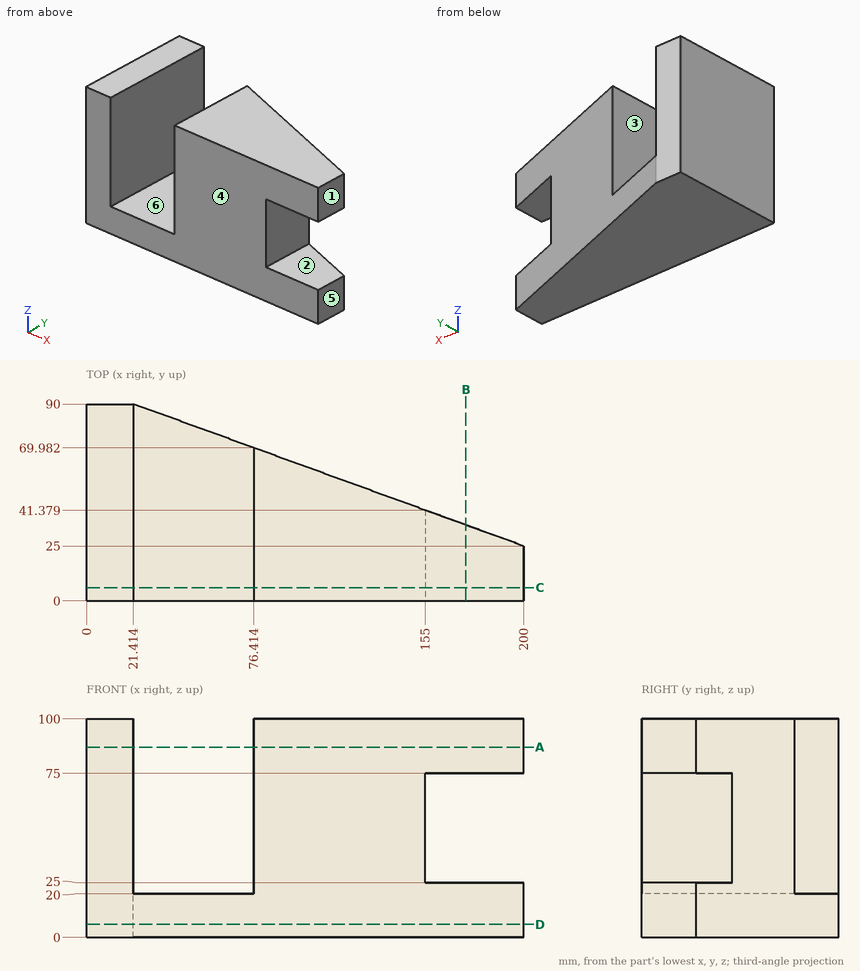
Here's the drawing with two shaded views (mm, measured from the low corner). I have some questions. A direction names the side the tool comes from. Coordinates: 2 decimals unless noted, no trailing zeros. Write each loop counter-clockwise with the first axis right and the second up, starting at its lowest first coordinate (ties: lowest second). Pieces come first, ordered by that corner, then holes.
Item 1: If I drill on line 1 (X direction, y = 8, z = 66); line 2 (Z direction, x = 162, y = 29.5); line 3 (Z direction, x = 45, y = 12.5), over which ranges is the centre line in solid material (lowest first)?
Item 2: I want a section at C-C on y = 6. Write out the boundary of the cut face in (x, z), and give its area (4 significant figures).
Item 3: If we mould it in two halves opening along X, with no side actions, what happens to the marked faces 4, 5 and 6? For each: +X half, -X half, draft (parallel to the pull), parting line (faces both ways), or undercut.
Item 4: I want a section at B-B on x = 173.5. Write out the boundary of the cut face in (y, z) (1 decimal).
Item 5: Will these pins go through, and if not, where does the flat tip stop? pin 1 (8 mm diameter, centred on x = 62, z = 20.5, fed in from +Y); pin 2 (12.5 mm diameter, centred on y = 19.5, z = 56, fed in from +X); pin 3 (5 mm diameter, centred on x = 66.5, y = 57.5, fed in from +Z).
Item 6: I want a section at A-A on z = 87. Write out the boundary of the cut face in (x, y), and give its area (3 significant figures).
Item 7: I want a section at D-D on z = 6. Write out the boundary of the cut face in (x, y), and give its area (3 significant figures).
Item 8: On a 3-axis mill with a long thin cutter (end or side, diameter ignored), from which of +Z, -Z, +X, -X, +Y, -Y can I reach the whole of each face in a straight line? I mean the marked faces 1, 2 and 3. Say none if no direction works.
Findings below:
1. line 1: x = 0 to 21.41, 76.41 to 155
1. line 2: z = 0 to 25, 75 to 100
1. line 3: z = 0 to 20
2. outline: (0, 0) - (200, 0) - (200, 25) - (155, 25) - (155, 75) - (200, 75) - (200, 100) - (76.41, 100) - (76.41, 20) - (21.41, 20) - (21.41, 100) - (0, 100) - close
2. area: 13,350 mm2
3. face 4: draft
3. face 5: +X half
3. face 6: undercut
4. outline: (0, 0) - (34.6, 0) - (34.6, 25) - (0, 25) - close; (0, 75) - (34.6, 75) - (34.6, 100) - (0, 100) - close
5. pin 1: stops at y = 76.67
5. pin 2: stops at x = 155
5. pin 3: stops at z = 20
6. outline: (0, 0) - (21.41, 0) - (21.41, 90) - (0, 90) - close; (76.41, 0) - (200, 0) - (200, 25) - (76.41, 69.98) - close
6. area: 7,800 mm2
7. outline: (0, 0) - (200, 0) - (200, 25) - (21.41, 90) - (0, 90) - close
7. area: 12,200 mm2
8. face 1: +Z, -Z, +X, +Y, -Y
8. face 2: +X, +Y, -Y
8. face 3: +Z, +Y, -Y
